Can you work these out from the model? Positions are in its coordinate system, mm. Face numbers are marked on the shaded views. Give positions to 0.01 mm unless a question says otherwise; leave off trailing zeros. Write each loop counter-clockwise with the first axis right and the second up, starting at its lowest first coordinate (ties: lowest second). Pieces come first, ordered by that corner, then holes.
1. Suppose I cut it at D-D (z = 8). Please give me the cut outline in (x, y).
2. If I drill on probe 1 along Z at (x, y) = (0, 18); probe 2 along Z at (x, y) = (0, 38); probe 3 along Y at (x, z) = (-12, 1.75), over which ranges is the centre line in solid material (lowest first)?
3. Suppose I cut it at C-C (y = 28). Please give me the cut outline in (x, z), and give its area (3 significant figures).
4. Suppose I cut it at B-B (x = 0). Please give me the cut outline in (y, z), and give its area (3 significant figures).
5. I'm going to push flat-ended pins straight in: pin 1 (4 mm diameter, centred on y = 6, z = 8, fed in from -X); pin 2 (1 mm diameter, centred on x = -3.5, y = 12, fed in from +Z); pin 3 (10 mm diameter, centred on y = 20, z = 1.5, fed in from -X). Where does each tip first touch, or does it pass through?
6. Suppose I cut it at A-A (z = 0). Please give me the cut outline in (x, y), and give its area (3 significant figures).
7. Thinking about a two-plate mould opening in X: for the marked faces 1, 2 and 3, which applies, pulls with the +X half, pulls with the -X half, needs draft (parallel to the pull), parting line crosses it, or undercut?
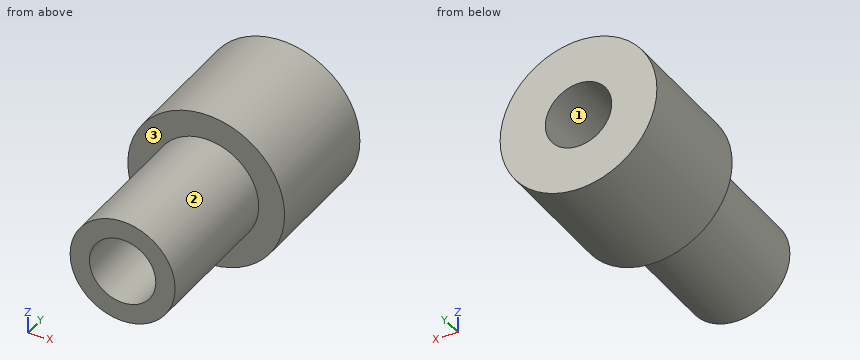
Autodesk Inventor part; units mm, degrees
ref_plane "YZ Plane" through (0, 0, 0) normal (1, 0, 0) x (0, 1, 0)
ref_plane "XZ Plane" through (0, 0, 0) normal (0, 1, 0) x (-1, 0, 0)
ref_plane "XY Plane" through (0, 0, 0) normal (0, 0, 1) x (1, 0, 0)
sketch "Sketch1" plane through (0, 0, 0) normal (0, 1, 0) x (-1, 0, 0)
  circle A0 centre (0, 0) radius 10.05
  dimension "d0" = 20.1
extrude "Extrusion1" add sketch "Sketch1" along normal blind 27.43
sketch "Sketch2" plane through (0, 27.43, 0) normal (0, 1, 0) x (1, 0, 0)
  circle A0 centre (0, 0) radius 15
  dimension "d3" = 30
extrude "Extrusion2" add sketch "Sketch2" along normal blind 24.7
thread "Thread1"
sketch "Sketch3" plane through (0, 0, 0) normal (0, -1, 0) x (1, 0, 0)
  circle A0 centre (0, 0) radius 6.35
  dimension "d8" = 12.7
extrude "Extrusion3" cut sketch "Sketch3" against normal blind 53
properties part number "AdaptadorMacho"
Checks:
1. outline: (-12.69, 27.43) - (-6.08, 27.43) - (-6.08, 0) - (6.08, 0) - (6.08, 27.43) - (12.69, 27.43) - (12.69, 52.13) - (-12.69, 52.13) - close
2. probe 1: z = -10.05 to -6.35, 6.35 to 10.05
2. probe 2: z = -15 to -6.35, 6.35 to 15
2. probe 3: y = 27.43 to 52.13
3. outline: circle Ø30 at (0, 0); hole circle Ø12.7 at (0, 0)
3. area: 580 mm2
4. outline: (0, -10.05) - (27.43, -10.05) - (27.43, -15) - (52.13, -15) - (52.13, -6.35) - (0, -6.35) - close; (0, 6.35) - (52.13, 6.35) - (52.13, 15) - (27.43, 15) - (27.43, 10.05) - (0, 10.05) - close
4. area: 630 mm2
5. pin 1: stops at x = -8.06
5. pin 2: stops at z = 9.59
5. pin 3: stops at x = -10.05
6. outline: (-15, 27.43) - (-10.05, 27.43) - (-10.05, 0) - (-6.35, 0) - (-6.35, 52.13) - (-15, 52.13) - close; (6.35, 0) - (10.05, 0) - (10.05, 27.43) - (15, 27.43) - (15, 52.13) - (6.35, 52.13) - close
6. area: 630 mm2
7. face 1: undercut
7. face 2: parting line crosses it
7. face 3: needs draft
